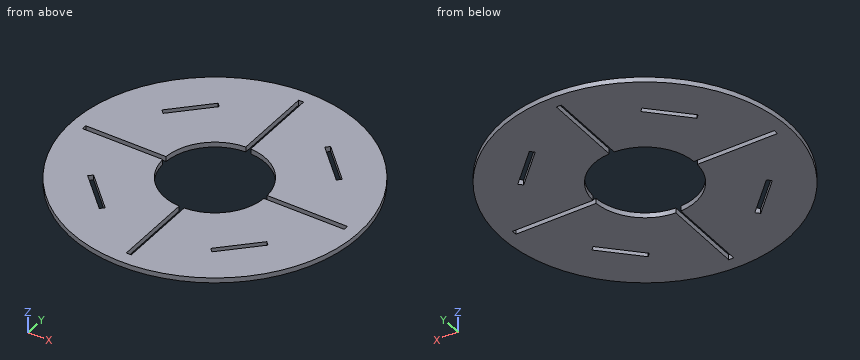
from build123d import *

# Parameters (mm, degrees)
SKETCH1_R           = 152.4
SKETCH1_R_2         = 53.721
BOSS_EXTRUDE1_DEPTH = 5.334
CUT_EXTRUDE2_REACH  = 217.592
CIRPATTERN1_COUNT   = 4
CUT_EXTRUDE3_REACH  = 217.592
CIRPATTERN2_COUNT   = 4


with BuildPart() as part:
    # Sketch1 → Boss-Extrude1 (new body)
    with BuildSketch(Plane.XY):
        Circle(SKETCH1_R)
        Circle(SKETCH1_R_2, mode=Mode.SUBTRACT)
    extrude(amount=BOSS_EXTRUDE1_DEPTH)

    # Sketch2 → Cut-Extrude2 (cut, up to next)
    with BuildSketch(Plane.XY.offset(5.334), mode=Mode.PRIVATE) as cut_extrude2_sk1:
        with BuildLine():
            Line((-2.6416, 53.656013553), (-2.6416, 138.746013553))
            Line((-2.6416, 138.746013553), (2.6416, 138.746013553))
            Line((2.6416, 138.746013553), (2.6416, 53.656013553))
            ThreePointArc((2.6416, 53.656013553), (0, 53.721), (-2.6416, 53.656013553))
        make_face()
    cut_extrude2_tool1 = extrude(cut_extrude2_sk1.sketch, amount=-CUT_EXTRUDE2_REACH, mode=Mode.PRIVATE) & part.part
    cut_extrude2 = cut_extrude2_tool1.solids().sort_by_distance((0, 96.222676, 5.334))[0]
    add(cut_extrude2, mode=Mode.SUBTRACT)

    # CirPattern1: Cut-Extrude2 ×4 about axis
    cirpattern1_axis = Axis((0, 0, 0), (0, 0, 1))
    for i in range(1, CIRPATTERN1_COUNT):
        add(cut_extrude2.rotate(cirpattern1_axis, i * 360 / CIRPATTERN1_COUNT), mode=Mode.SUBTRACT)

    # Sketch3 → Cut-Extrude3 (cut, up to next)
    with BuildSketch(Plane.XY.offset(5.334), mode=Mode.PRIVATE) as cut_extrude3_sk1:
        Polygon((-95.639727689, 59.718703205), (-59.718703205, 95.639727689), (-55.946995634, 91.868020119), (-91.868020119, 55.946995634), align=None)
    cut_extrude3_tool1 = extrude(cut_extrude3_sk1.sketch, amount=-CUT_EXTRUDE3_REACH, mode=Mode.PRIVATE) & part.part
    cut_extrude3 = cut_extrude3_tool1.solids().sort_by_distance((-75.793362, 75.793362, 5.334))[0]
    add(cut_extrude3, mode=Mode.SUBTRACT)

    # CirPattern2: Cut-Extrude3 ×4 about axis
    cirpattern2_axis = Axis((0, 0, 0), (0, 0, 1))
    for i in range(1, CIRPATTERN2_COUNT):
        add(cut_extrude3.rotate(cirpattern2_axis, i * 360 / CIRPATTERN2_COUNT), mode=Mode.SUBTRACT)


solid = part.part
Could you check a few things on this model? Use its own coordinates, in mm. Give positions to 0.01 mm unless a question says otherwise; leave off trailing zeros. Loops run counter-clockwise (first coordinate to the right, second up) from the corner with the lowest first, then second, coordinate; pieces in that order, holes last. Notation, with made-up numbers: M 58.25,68.5 L 72.25,68.5 A34 cw 72.25,100.5 Z; hole C 76.25,83 d7. An arc over 180 degrees is marked long. Answer as a JSON object with one key per item and string values.
Q1. Suppose I cut it at A-A, the plane z = 0.85. State how many separate pieces and enclosed holes the cut face has, plus the area to 3 significant figures.
Values found:
{"separate pieces": "1", "enclosed holes": "5", "area": "61,000 mm²"}
Q2. Suppose I cut it at D-D, the plane x = 10.5. List the corners of the cut face in (y, z) for me, plus the area to 3 significant figures.
Values found:
{"outline": "M -152.04,0 L -52.68,0 L -52.68,5.33 L -152.04,5.33 Z; M 52.68,0 L 152.04,0 L 152.04,5.33 L 52.68,5.33 Z", "area": "1,060 mm²"}
Q3. For P1, Ø3, axis at x = -86, z = 1.5, coming from the -Y side; P2, Ø2, axis at x = 25.5, z = 1.5, coming from the -Y side; P3, Ø1.6, axis at x = 85, z = 2, coming from the -Y side, each with a flat end and sliding along its axis, tell me the tip position at first contact or that it passes through.
Values found:
{"P1": "stops at y = -126.83", "P2": "stops at y = -150.42", "P3": "stops at y = -127.03"}
Q4. If I drill on probe 1 along Y at (x, z) = (75, 3.35); probe 2 along X at (y, z) = (-85, 2.4); probe 3 along X at (y, z) = (1, 0.6), over which ranges is the centre line in solid material (lowest first)? Write a range as [from, to].
Values found:
{"probe 1": "y = [-132.67, -80.36], [-72.82, -2.64], [2.64, 72.82], [80.36, 132.67]", "probe 2": "x = [-126.49, -70.36], [-62.82, -2.64], [2.64, 62.82], [70.36, 126.49]", "probe 3": "x = [-152.4, -138.75], [138.75, 152.4]"}
Q5. Suppose I cut it at B-B, the plane x = 64. List the corners of the cut face in (y, z) for me, plus the area to 3 significant figures.
Values found:
{"outline": "M -138.31,0 L -91.36,0 L -91.36,5.33 L -138.31,5.33 Z; M -83.82,0 L -2.64,0 L -2.64,5.33 L -83.82,5.33 Z; M 2.64,0 L 83.82,0 L 83.82,5.33 L 2.64,5.33 Z; M 91.36,0 L 138.31,0 L 138.31,5.33 L 91.36,5.33 Z", "area": "1,370 mm²"}
Q6. Suppose I cut it at C-C, the plane y = -86. List the corners of the cut face in (x, z) for me.
Values found:
{"outline": "M -125.82,0 L -69.36,0 L -69.36,5.33 L -125.82,5.33 Z; M -61.82,0 L -2.64,0 L -2.64,5.33 L -61.82,5.33 Z; M 2.64,0 L 61.82,0 L 61.82,5.33 L 2.64,5.33 Z; M 69.36,0 L 125.82,0 L 125.82,5.33 L 69.36,5.33 Z"}
